Can you work these out from the model? Positions are in its coordinate system, mm. Round coordinates to 2 decimals unless told otherwise and drop trailing zeros. Loops run counter-clockwise (first coordinate to the right, second up) from the corner with the lowest first, then second, coordinate; pieces in that order, holes last. Notation, with made-up numbers: (34, 87) -> (75, 87) arc R8 cw to (75, 91) -> close; hole circle Ø9 at (30, 62). An arc over 180 degrees is marked (long way). Answer as a JSON object with one key per item and string values.
Autodesk Inventor part; units mm, degrees
ref_plane "Work Plane1" through (-152.4, 0, 0) normal (1, 0, 0) x (0, 0, -1)
ref_plane "YZ Plane" through (0, 0, 0) normal (1, 0, 0) x (0, 1, 0)
ref_plane "XZ Plane" through (0, 0, 0) normal (0, 1, 0) x (-1, 0, 0)
sketch "Sketch1" plane through (0, 0, 0) normal (0, 1, 0) x (-1, 0, 0)
  line L0 (0, 0) -> (304.8, 0)
  line L1 (304.8, 0) -> (304.8, -25.4)
  line L2 (304.8, -25.4) -> (0, -25.4)
  line L3 (0, -25.4) -> (0, 0)
  dimension "d0" = 304.8
  dimension "d1" = 25.4
extrude "Extrusion1" add sketch "Sketch1" along normal blind 25.4
hole "Hole1" at (-292.1, 25.4, -12.7) direction (0, -1, 0) diameter 6.35 end through all
ref_plane "Work Plane1" through (-152.4, 0, 0) normal (1, 0, 0) x (0, 0, -1)
mirror "Mirror1" about plane through (-152.4, 0, 0) normal (1, 0, 0) of "Hole1"
fillet "Fillet1" radius 12.7 4 edges at (-304.8, 12.7, -25.4) (-304.8, 12.7, 0) (0, 12.7, -25.4) (0, 12.7, 0)
chamfer "Chamfer1" distance 2.54 angle 45 8 edges at (-152.4, 25.4, 0) (-3.7197, 25.4, -21.6803) (-152.4, 25.4, -25.4) (-301.0803, 25.4, -21.6803) (-152.4, 0, 0) (-301.0803, 0, -21.6803) (-152.4, 0, -25.4) (-3.7197, 0, -21.6803)
properties part number "longerBar"
Q1. I want a section at B-B, the plane x = -60.5. Write out the boundary of the cut face in (y, z).
Determined:
{"outline": "(0, -22.86) -> (2.54, -25.4) -> (22.86, -25.4) -> (25.4, -22.86) -> (25.4, -2.54) -> (22.86, 0) -> (2.54, 0) -> (0, -2.54) -> close"}
Q2. I want a section at A-A, the plane y = 16.25. Give the number of separate pieces and of enclosed holes in the cut face, then the cut area to 3 significant figures.
Determined:
{"separate pieces": "1", "enclosed holes": "2", "area": "7,540 mm²"}
Q3. We'd pull the mould along X, two halves only. Please class faces 1 (the cylindrical face through (-301.18, 12.84, -3.82)), 2 (the cylindrical face through (-295.25, 12.52, -13.11)), 3 (the cylindrical face through (-9.9, 12.5, -11.2)), 4 (the conical face through (-5.089, 24.677, -20.48)): pulls with the +X half, pulls with the -X half, needs draft (parallel to the pull), parting line crosses it, or undercut.
Determined:
{"face 1": "pulls with the -X half", "face 2": "undercut", "face 3": "undercut", "face 4": "pulls with the +X half"}
Q4. I'm going to push flat-ended pins straight in: pin 1 (5.5 mm diameter, centred on x = -12.7, z = -12.7, fed in from -Y); pin 2 (2 mm diameter, centred on y = 17, z = -17, fed in from +X). Where does each tip first touch, or does it pass through?
Determined:
{"pin 1": "through", "pin 2": "x = -0.44"}
Q5. If I drill on L1, parallel to X at y = 9.5, z = -12.7 (3 decimals); L2, parallel to Z at x = -292.1, y = 16.25 (3 decimals); L3, parallel to X at y = 17, z = -11.25, over which ranges is the centre line in solid material (lowest first)? Write a range as [from, to].
Determined:
{"L1": "[-304.8, -295.275], [-288.925, -15.875], [-9.525, 0]", "L2": "[-25.4, -15.875], [-9.525, 0]", "L3": "[-304.72, -294.92], [-289.28, -15.52], [-9.88, -0.08]"}
